Can you work these out from the drawing? Everything is in mm from the part's minimum corner. A direction names the side the tool comes from. Round coordinates to 2 decimals unless told otherwise and drop trailing zeros. Write each loop counter-clockwise with the first axis right and the second up, starting at its lowest first coordinate (ties: lowest second). Pieces come first, ordered by that corner, then holes.
Q1. For the marked faces 1, 2 and 3, which set-ups out of +Z, -Z, +X, -X, +Y, -Y let a thin tool reach every point of the face, with its end or its side?
Q2. If we section it at C-C (y = 13): Please give me the cut outline in (x, z).
Q3. If we section it at B-B (x = 15): Please give me the cut outline in (y, z) (1 decimal), plus the area to 3 significant figures.
Q4. Please list where these lines run through material, in increasing order: line 1 along Y through (x, z) = (10.5, 2.8); line 2 along X through (y, z) = (2, 1.2); line 3 along X through (y, z) = (9, 2.2).
Q5. If we section it at A-A (z = 1.35): Please give me the cut outline in (x, y).
Q6. I'm going to push a flat-ended pin straight in: pin 1 Ø1 at (x, z) = (16.5, 2) entering from -Y. Where does the tip first touch, or does it pass through?
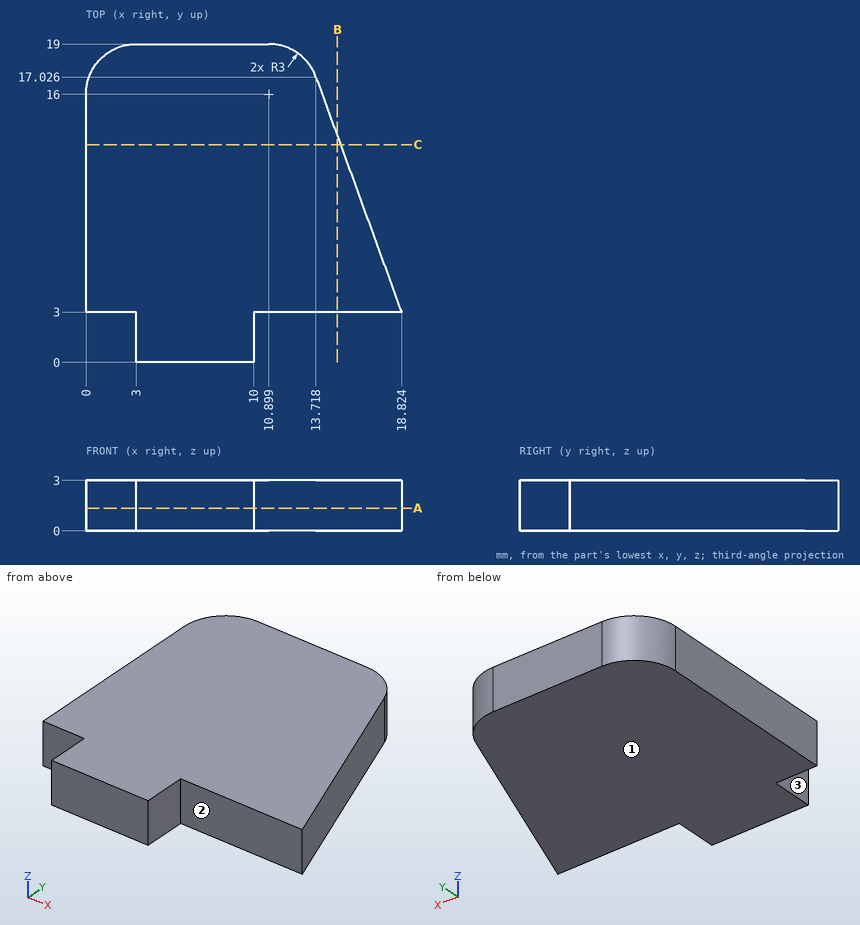
A:
1. face 1: -Z, +X, -X, +Y, -Y
1. face 2: +Z, -Z, +X, -Y
1. face 3: +Z, -Z, -X, -Y
2. outline: (0, 0) - (15.18, 0) - (15.18, 3) - (0, 3) - close
3. outline: (3, 0) - (13.5, 0) - (13.5, 3) - (3, 3) - close
3. area: 31.5 mm2
4. line 1: y = 3 to 19
4. line 2: x = 3 to 10
4. line 3: x = 0 to 16.64
5. outline: (0, 3) - (3, 3) - (3, 0) - (10, 0) - (10, 3) - (18.82, 3) - (13.72, 17.03) arc R3 ccw to (10.9, 19) - (3, 19) arc R3 ccw to (0, 16) - close
6. pin 1: stops at y = 3
